Geometry: final body of the model. Coordinates: model frame, mm. Round coordinates to 2 decimals unless told otherwise and drop trailing zeros. Loops run counter-clockwise (first coordinate to the right, second up) from the corner with the lowest first, then second, coordinate; pieces in that order, holes last. Notation, with made-up numbers: (-10.75, 18) - (26.25, 18) arc R21 ccw to (26.25, 41) - close; hole circle Ø4 at (89.25, 70). An arc over 180 degrees is marked (long way). Write item = value, one per line. Start each with the question number.
Item 1: Draft query along Y for faces 1 (the flat face through (175, 3, 5)), 2 (the cylindrical face through (175, 0, 2)). Return one class per face: pulls with the +Y half, pulls with the -Y half, needs draft (parallel to the pull), parting line crosses it, or undercut.
Item 2: Section D-D (x = -45.5). Return loops of the section in (y, z).
Item 3: First-contact query: pin 1 (11.5 mm diameter, centred on x = 180, y = 0, fed in from +Z); pin 2 (9 mm diameter, centred on x = 0, y = -180, fed in from -Z). Flat tips, straight axial feed; report the tip coordinate or a pass-through.
Item 4: Section C-C (z = 3.9). Return loops of the section in (x, y), plus the area to 3 significant figures.
Item 5: Section A-A (y = 0). Return loops of the section in (x, z), plus the area to 3 significant figures.
Item 6: Line query: line 1 (Y direction, x = 0, z = 4); line 2 (X direction, y = -125.5, z = 4.75); line 3 (Y direction, x = 180, z = 3.45). Output: solid intervals per line, ascending. Write a range as from..to.
from build123d import *

# Parameters (mm, degrees)
F0_W     = 400
F0_H     = 400
F0_R     = 5
F0_W_2   = 320
F0_H_2   = 320
F1_DEPTH = 5


with BuildPart() as f1:
    # F0 (on Top) → F1 (new body)
    with BuildSketch(Plane.XY):
        Rectangle(F0_W, F0_H)
        with Locations((0, -180)):
            Circle(F0_R, mode=Mode.SUBTRACT)
        with Locations((-180, 0)):
            Circle(F0_R, mode=Mode.SUBTRACT)
        Rectangle(F0_W_2, F0_H_2, mode=Mode.SUBTRACT)
        with Locations((180, 0)):
            Circle(F0_R, mode=Mode.SUBTRACT)
        with Locations((0, 180)):
            Circle(F0_R, mode=Mode.SUBTRACT)
    extrude(amount=F1_DEPTH)


solid = f1.part
Taken from the geometry:
q1.face_1 = needs draft
q1.face_2 = undercut
q2.outline = (-200, 0) - (-160, 0) - (-160, 5) - (-200, 5) - close; (160, 0) - (200, 0) - (200, 5) - (160, 5) - close
q3.pin_1 = 5
q3.pin_2 = through
q4.outline = (-200, -200) - (200, -200) - (200, 200) - (-200, 200) - close; hole circle Ø10 at (-180, 0); hole (-160, -160) - (160, -160) - (160, 160) - (-160, 160) - close; hole circle Ø10 at (0, -180); hole circle Ø10 at (0, 180); hole circle Ø10 at (180, 0)
q4.area = 57,300 mm^2
q5.outline = (-200, 0) - (-185, 0) - (-185, 5) - (-200, 5) - close; (-175, 0) - (-160, 0) - (-160, 5) - (-175, 5) - close; (160, 0) - (175, 0) - (175, 5) - (160, 5) - close; (185, 0) - (200, 0) - (200, 5) - (185, 5) - close
q5.area = 300 mm^2
q6.line_1 = -200..-185, -175..-160, 160..175, 185..200
q6.line_2 = -200..-160, 160..200
q6.line_3 = -200..-5, 5..200
